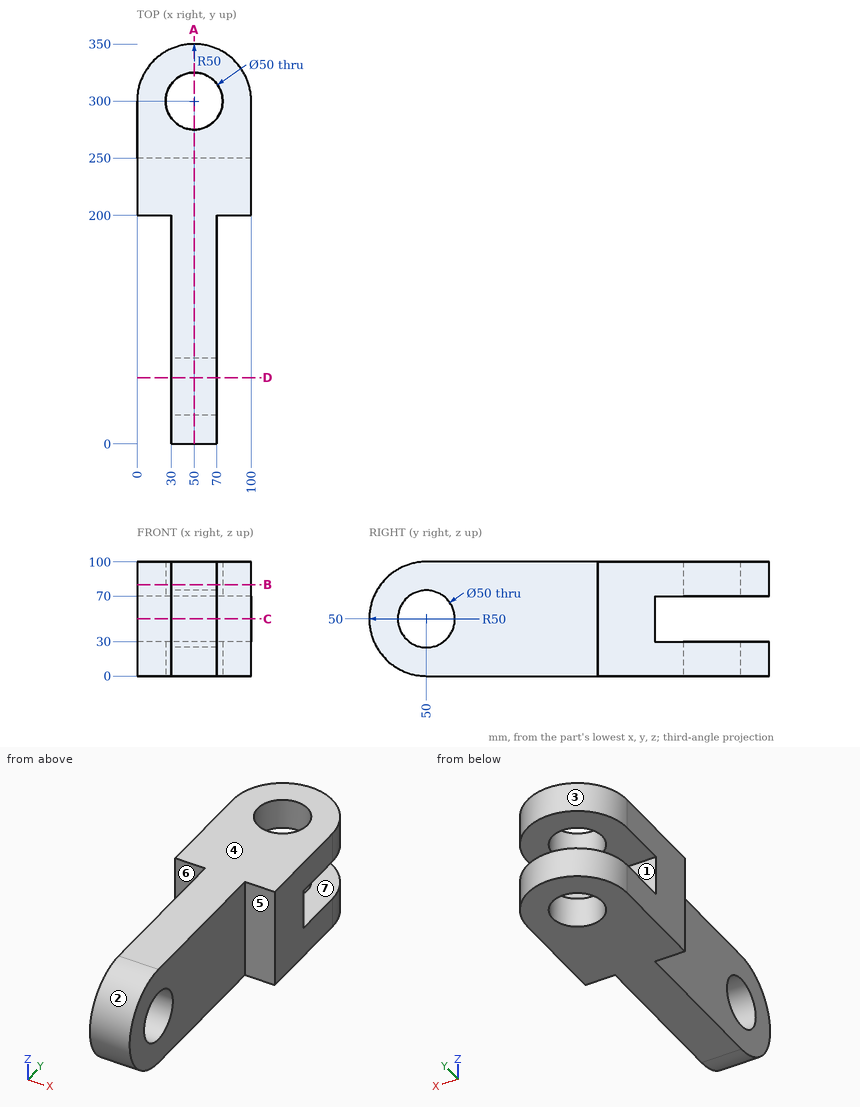
Study the drawing (mm; zero at the part's minimum x, y, z) and answer. A direction names the side the tool comes from. Give positions to 0.01 mm unless a question says otherwise; leave off trailing zeros. Write each loop counter-clockwise with the first axis right and the second up, starting at its lowest first coordinate (ties: lowest second). Pieces come first, ordered by that corner, then holes. Notation, with made-up numbers: (75, -17) - (84, -17) arc R17 ccw to (84, -9) - close; hole circle Ø8 at (35.25, 41.5). An arc over 180 degrees is marked (long way). Use a Markdown table: item, result.
1. For a pull along Z with two mould halves and no side action, classify the marked faces 1, 2 and 3 as released by +Z, released by -Z, zero draft, split by the parting line, or undercut.
Values follow:
| item | result |
|---|---|
| face 1 | undercut |
| face 2 | split by the parting line |
| face 3 | zero draft |
2. Section A-A on x = 50 is taken. Write down the section's boundary in (y, z).
Values follow:
| item | result |
|---|---|
| outline | (50, 0) - (275, 0) - (275, 30) - (250, 30) - (250, 70) - (275, 70) - (275, 100) - (50, 100) arc R50 ccw to start; (325, 0) - (350, 0) - (350, 30) - (325, 30) - close; (325, 70) - (350, 70) - (350, 100) - (325, 100) - close; hole circle Ø50 at (50, 50) |
3. Section B-B on z = 80 is taken. Write down the section's boundary in (x, y).
Values follow:
| item | result |
|---|---|
| outline | (0, 200) - (30, 200) - (30, 10) - (70, 10) - (70, 200) - (100, 200) - (100, 300) arc R50 ccw to (0, 300) - close; hole circle Ø50 at (50, 300) |
4. Find the intervals of material crossed by probe 1 along Z at (x, y) = (93, 261); probe 2 along Y at (x, z) = (56, 50); probe 3 along X at (y, z) = (300, 78), in increasing order. Write a range as from..to.
Values follow:
| item | result |
|---|---|
| probe 1 | z = 0..30, 70..100 |
| probe 2 | y = 0..25, 75..250 |
| probe 3 | x = 0..25, 75..100 |
5. Section D-D on y = 58 is taken. Write down the section's boundary in (x, z).
Values follow:
| item | result |
|---|---|
| outline | (30, 0) - (70, 0) - (70, 26.31) - (30, 26.31) - close; (30, 73.69) - (70, 73.69) - (70, 100) - (30, 100) - close |
6. Each of these flat-tipped pins is pushed along its axis until it touches: P1, Ø1.5, axis at x = 56.5, z = 55, coming from the +Y side; P2, Ø8, axis at y = 52, z = 76.5, coming from the +X side; P3, Ø15, axis at x = 78, z = 28, coming from the -Y side. Where does it stop, or does it pass through?
Values follow:
| item | result |
|---|---|
| P1 | stops at y = 250 |
| P2 | stops at x = 70 |
| P3 | stops at y = 200 |
7. A tool of negligible diameter and unlimited length cuts with its end or side. For the marked faces 4, 5, 6 and 7, from which of +Z, -Z, +X, -X, +Y, -Y can it reach the whole face along a straight path? Write none if from no direction.
Values follow:
| item | result |
|---|---|
| face 4 | +Z, +X, -X, +Y, -Y |
| face 5 | +Z, -Z, +X, -Y |
| face 6 | +Z, -Z, -X, -Y |
| face 7 | +X, -X, +Y |
8. Section C-C on z = 50 is taken. Write down the section's boundary in (x, y), plus the area to 3 significant figures.
Values follow:
| item | result |
|---|---|
| outline | (0, 200) - (30, 200) - (30, 75) - (70, 75) - (70, 200) - (100, 200) - (100, 250) - (0, 250) - close; (30, 0) - (70, 0) - (70, 25) - (30, 25) - close |
| area | 11,000 mm² |
